Design review of the part built by this model. Coordinates are the model's own, in mm. A direction names the side the tool comes from. Coordinates: 2 decimals unless noted, no trailing zeros. Write each loop counter-clockwise with the first axis right and the second up, starting at its lowest first coordinate (ties: lowest second). Pieces come first, ordered by that corner, then holes. Notation, with made-up numbers: (78.25, -7) -> (88.25, -7) arc R20 ccw to (88.25, 31) -> close; hole circle Ø7 at (73, -27.75). An arc over 180 degrees is marked (long way). Write item = value, one per line. Start each with the question number.
```python
from build123d import *

# Parameters (mm, degrees)
SKETCH_2_R      = 1.55
SKETCH_2_R_2    = 1.384923923
EXTRUDE_1_DEPTH = 2.5


with BuildPart() as part:
    # 草图2 → 凸台-拉伸1 (new body)
    # profile 1 of 3: a face of its own
    with BuildSketch(Plane.XY):
        with BuildLine():
            Line((-22.577164466, 18.92268553), (-22.577164466, -18.92268553))
            ThreePointArc((-22.577164466, -18.92268553), (-27.577164466, -23.92268553), (-32.577164466, -18.92268553))
            Line((-32.577164466, -18.92268553), (-32.577164466, 18.92268553))
            ThreePointArc((-32.577164466, 18.92268553), (-27.577164466, 23.92268553), (-22.577164466, 18.92268553))
        make_face()
        with Locations((-27.577164466, -18.92268553)):
            Circle(SKETCH_2_R, mode=Mode.SUBTRACT)
        with Locations((-27.577164466, 18.92268553)):
            Circle(SKETCH_2_R, mode=Mode.SUBTRACT)
    # profile 2 of 3: a face of its own
    with BuildSketch(Plane.XY):
        with BuildLine():
            Line((22.577164466, 18.92268553), (22.577164466, -18.92268553))
            ThreePointArc((22.577164466, -18.92268553), (27.577164466, -23.92268553), (32.577164466, -18.92268553))
            Line((32.577164466, -18.92268553), (32.577164466, 18.92268553))
            ThreePointArc((32.577164466, 18.92268553), (27.577164466, 23.92268553), (22.577164466, 18.92268553))
        make_face()
        with Locations((27.577164466, -18.92268553)):
            Circle(SKETCH_2_R, mode=Mode.SUBTRACT)
        with Locations((27.577164466, 18.92268553)):
            Circle(SKETCH_2_R, mode=Mode.SUBTRACT)
    # profile 3 of 3: a face of its own
    with BuildSketch(Plane.XY):
        with BuildLine():
            Line((-22.5, 5), (22.5, 5))
            ThreePointArc((22.5, 5), (27.5, 0), (22.5, -5))
            Line((22.5, -5), (-22.5, -5))
            ThreePointArc((-22.5, -5), (-27.5, 0), (-22.5, 5))
        make_face()
        with Locations((-22.5, 0)):
            Circle(SKETCH_2_R_2, mode=Mode.SUBTRACT)
        with Locations((22.5, 0)):
            Circle(SKETCH_2_R_2, mode=Mode.SUBTRACT)
    extrude(amount=EXTRUDE_1_DEPTH)


solid = part.part
```
(1) Take a section at B-B, the plane z = 0.4. State the section outline as (x, y) points, then the cut area to 3 significant figures.
(2) Mouldability with a two-part tool opening along Y and no side actions: class faces 1 (the face through (-22.577, -12, 1)), 2 (the face through (27.69, 23.92, 1.23)), 3 (the face through (0, -5, 1)), 4 (the face through (22.577, 0, 1)) as pulls with the +Y half, pulls with the -Y half, needs draft (parallel to the pull), parting line crosses it, or undercut.
(3) For line 1 (X direction, y = 8, z = 0.3); line 2 (X direction, y = -19.5, z = 0.2); line 3 (X direction, y = -18.5, z = 1.65), list the stretches that pass through material, from the lowest coordinate up.
(4) For faces 5 (the face through (-21.115, -0.032, 1.232)), 6 (the face through (-22.577, 12, 1)), 7 (the face through (32.577, 0, 1)), 8 (the face through (-32.577, 0, 1)), 9 (the face through (22.577, -12, 1)), list the 3-axis set-ups (+Z, -Z, +X, -X, +Y, -Y) from which the entire face can be reached by the end or side of a thin tool; tool diameter is ignored.
(5) Take a section at D-D, the plane x = -14. State the section outline as (y, z) points, then the cut area to 3 significant figures.
(6) For pin 1 Ø1.9 at (x, y) = (-27.58, -18.92) entering from +Z; pin 2 Ø0.8 at (x, z) = (2.5, 1) entering from +Y; pin 3 Ø1.2 at (x, z) = (2.5, 1.5) entering from -Y, all flat-tipped, find the tip position at first contact; note any pin that passes through.
(7) Take a section at A-A, the plane y = 0. State the section outline as (x, z) points, then the cut area to 3 significant figures.
(8) Take a section at C-C, the plane y = 6.5. State the section outline as (x, z) points.
Report:
q1.outline = (-32.58, -18.92) arc R5 ccw to (-22.58, -18.92) -> (-22.58, -5) arc R5 ccw to (-22.5, -5) -> (22.5, -5) arc R5 ccw to (22.58, -5) -> (22.58, -18.92) arc R5 ccw to (32.58, -18.92) -> (32.58, 18.92) arc R5 ccw to (22.58, 18.92) -> (22.58, 5) arc R5 ccw to (22.5, 5) -> (-22.5, 5) arc R5 ccw to (-22.58, 5) -> (-22.58, 18.92) arc R5 ccw to (-32.58, 18.92) -> close; hole circle Ø3.1 at (-27.58, -18.92); hole circle Ø3.1 at (-27.58, 18.92); hole (-22.58, -1.38) arc R1.38 ccw (long way) to (-22.58, 1.38) -> close; hole (22.58, -1.38) -> (22.58, 1.38) arc R1.38 ccw (long way) to start; hole circle Ø3.1 at (27.58, -18.92); hole circle Ø3.1 at (27.58, 18.92)
q1.area = 1,330 mm2
q2.face_1 = needs draft
q2.face_2 = pulls with the +Y half
q2.face_3 = pulls with the -Y half
q2.face_4 = undercut
q3.line_1 = -32.58 to -22.58, 22.58 to 32.58
q3.line_2 = -32.54 to -29.02, -26.14 to -22.61, 22.61 to 26.14, 29.02 to 32.54
q3.line_3 = -32.58 to -29.07, -26.09 to -22.58, 22.58 to 26.09, 29.07 to 32.58
q4.face_5 = +Z, -Z
q4.face_6 = +Z, -Z, +Y
q4.face_7 = +Z, -Z, +X, +Y, -Y
q4.face_8 = +Z, -Z, -X, +Y, -Y
q4.face_9 = +Z, -Z, -Y
q5.outline = (-5, 0) -> (5, 0) -> (5, 2.5) -> (-5, 2.5) -> close
q5.area = 25.0 mm2
q6.pin_1 = through
q6.pin_2 = 5
q6.pin_3 = -5
q7.outline = (-32.58, 0) -> (-22.58, 0) -> (-22.58, 2.5) -> (-32.58, 2.5) -> close; (-21.12, 0) -> (21.12, 0) -> (21.12, 2.5) -> (-21.12, 2.5) -> close; (22.58, 0) -> (32.58, 0) -> (32.58, 2.5) -> (22.58, 2.5) -> close
q7.area = 156 mm2
q8.outline = (-32.58, 0) -> (-22.58, 0) -> (-22.58, 2.5) -> (-32.58, 2.5) -> close; (22.58, 0) -> (32.58, 0) -> (32.58, 2.5) -> (22.58, 2.5) -> close
